The model under review builds one solid part; all positions refer to its coordinate system, in mm. Face numbers are marked on the shaded views. A direction names the side the tool comes from. Give positions to 0.01 mm unless a question says otherwise; leave off trailing zeros. One line per item, written item: value. Start each with the question number.
Q1. To check wall thickness, follow line 1 along Y through (x, z) = (4.25, 0); line 2 along Y through (x, z) = (1.2, 0); line 3 along X through (y, z) = (-3, -15.5). State the ranges of each line that lie inside material, in increasing order. Write a range as from..to.
Q2. For the marked faces 1, 2 and 3, list the 3-axis set-ups (+Z, -Z, +X, -X, +Y, -Y) from which the entire face can be reached by the end or side of a thin tool; tool diameter is ignored.
Q3. For pin 1 (1.6 mm diameter, centred on x = 19, y = 5.5, fed in from +Z); pin 2 (4 mm diameter, centred on x = 4, z = -2.5, fed in from +Y); pin 3 (13.5 mm diameter, centred on y = 27.5, z = 0, fed in from +X), all flat-tipped, find the tip position at first contact; note any pin that passes through.
Q4. Mouldability with a two-part tool opening along Y and no side actions: class the marked faces 4, 5 and 6 as released by +Y, released by -Y, zero draft, split by the parting line, or undercut.
Q5. We need section A-A on z = 0. Give the number of separate pieces and of enclosed holes in the cut face, plus the area to 3 significant figures.
```python
from build123d import *

# Parameters (mm, degrees)
SKETCH_2_R          = 4.2
CUT_EXTRUDE_1_DEPTH = 62.846584384
SKETCH_3_R          = 4.5
CUT_EXTRUDE_2_DEPTH = 62.846584384
SKETCH_5_W          = 4
SKETCH_5_H          = 4
CUT_EXTRUDE_3_DEPTH = 62.846584384
FILLET_1_R          = 0.2
CHAMFER_1_SIZE      = 1
CHAMFER_2_SIZE      = 0.5


with BuildPart() as part:
    # Эскиз1 → Повернуть1 (revolve)
    with BuildSketch(Plane.XY, mode=Mode.PRIVATE) as revolve_1_sk:
        Polygon((0, 12.5), (0, 40), (8, 40), (8, 9), (25, 9), (25, 5.5), (2, 5.5), (2, 12.5), align=None)
    revolve(revolve_1_sk.sketch.rotate(Axis((0, 0, 0), (1, 0, 0)), 90), axis=Axis((0, 0, 0), (1, 0, 0)))

    # Эскиз2 → Вырез-Вытянуть1 (cut, through all)
    with BuildSketch(Plane(origin=(0, 0, 0), x_dir=(0, 0, -1), z_dir=(1, 0, 0))):
        with Locations(Location((0, 27.5, 0), (0, 0, 180))):
            Circle(SKETCH_2_R)
    extrude(amount=CUT_EXTRUDE_1_DEPTH, mode=Mode.SUBTRACT)

    # Эскиз3 → Вырез-Вытянуть2 (cut, through all)
    with BuildSketch(Plane(origin=(0, 0, 0), x_dir=(0, 0, -1), z_dir=(1, 0, 0))):
        with Locations(Location((0, -27.5, 0), (0, 0, 180))):
            Circle(SKETCH_3_R)
    extrude(amount=CUT_EXTRUDE_2_DEPTH, mode=Mode.SUBTRACT)

    # Эскиз5 → Вырез-Вытянуть3 (cut, through all)
    with BuildSketch(Plane(origin=(0, 0, 0), x_dir=(0, 0, -1), z_dir=(1, 0, 0))):
        with Locations((0, 5.3)):
            Rectangle(SKETCH_5_W, SKETCH_5_H)
    extrude(amount=CUT_EXTRUDE_3_DEPTH, mode=Mode.SUBTRACT)

    # Скругление1
    fillet_1_edges = [part.edges().sort_by_distance(p)[0] for p in [
        (13.5, 7.3, -2),
        (13.5, 7.3, 2),
    ]]
    fillet(fillet_1_edges, radius=FILLET_1_R)

    # Фаска1
    chamfer_1_edges = [part.edges().sort_by_distance(p)[0] for p in [
        (25, -5.5, 0),
        (25, 0, -9),
        (8, 0, -40),
        (0, 0, -40),
    ]]
    chamfer(chamfer_1_edges, length=CHAMFER_1_SIZE)

    # Фаска2
    chamfer_2_edges = [part.edges().sort_by_distance(p)[0] for p in [
        (8, 27.5, -4.2),
        (8, -27.5, -4.5),
    ]]
    chamfer(chamfer_2_edges, length=CHAMFER_2_SIZE)


solid = part.part
```
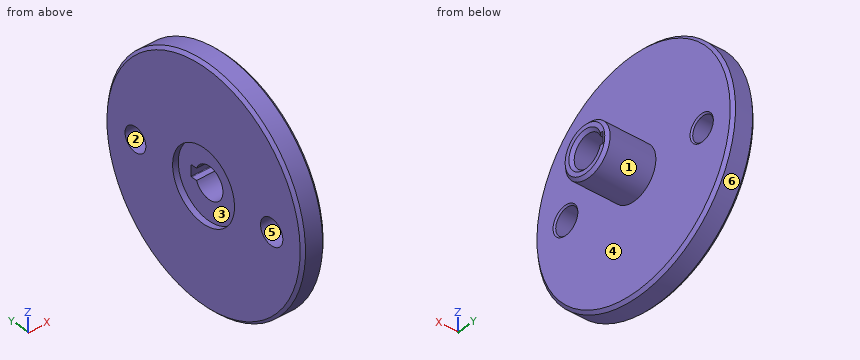
Solved:
1. line 1: -40..-32, -23..-5.5, 7.3..23.3, 31.7..40
1. line 2: -40..-32, -23..-12.5, 12.5..23.3, 31.7..40
1. line 3: 0..8
2. face 1: +X
2. face 2: +X, -X
2. face 3: -X
3. pin 1: z = 7.68
3. pin 2: y = 40
3. pin 3: x = 8
4. face 4: zero draft
4. face 5: undercut
4. face 6: split by the parting line
5. separate pieces: 4
5. enclosed holes: 0
5. area: 458 mm2
